```python
from build123d import *

# Parameters (mm, degrees)
EXTRUDE_1_DEPTH     = 15.5
EXTRUDE_2_DEPTH     = 3
FILLET_2_R          = 2
SKETCH_4_W          = 3
SKETCH_4_H          = 70
EXTRUDE_3_DEPTH     = 4
FILLET_3_R          = 1.5
CUT_EXTRUDE_3_DEPTH = 151.652746407
SKETCH_10_R         = 1.75
CUT_EXTRUDE_4_DEPTH = 164.099662783
SKETCH_9_R          = 1.75
CUT_EXTRUDE_5_DEPTH = 164.099662783


with BuildPart() as part:
    # 草图1 → 凸台-拉伸1 (new body)
    with BuildSketch(Plane(origin=(0, 0, 0), x_dir=(1, 0, 0), z_dir=(0, 1, 0))):
        with BuildLine():
            Line((-115, 85), (115, 85))
            ThreePointArc((115, 85), (118.535533906, 83.535533906), (120, 80))
            Line((120, 80), (120, -80))
            ThreePointArc((120, -80), (118.535533906, -83.535533906), (115, -85))
            Line((115, -85), (-115, -85))
            ThreePointArc((-115, -85), (-118.535533906, -83.535533906), (-120, -80))
            Line((-120, -80), (-120, 80))
            ThreePointArc((-120, 80), (-118.535533906, 83.535533906), (-115, 85))
        make_face()
        with BuildLine():
            Line((-112.5, 82.5), (112.5, 82.5))
            ThreePointArc((112.5, 82.5), (116.035533906, 81.035533906), (117.5, 77.5))
            Line((117.5, 77.5), (117.5, -77.5))
            ThreePointArc((117.5, -77.5), (116.035533906, -81.035533906), (112.5, -82.5))
            Line((112.5, -82.5), (-112.5, -82.5))
            ThreePointArc((-112.5, -82.5), (-116.035533906, -81.035533906), (-117.5, -77.5))
            Line((-117.5, -77.5), (-117.5, 77.5))
            ThreePointArc((-117.5, 77.5), (-116.035533906, 81.035533906), (-112.5, 82.5))
        make_face(mode=Mode.SUBTRACT)
    extrude(amount=EXTRUDE_1_DEPTH)

    # 草图3 → 凸台-拉伸2 (add)
    with BuildSketch(Plane(origin=(0, 15.5, 0), x_dir=(1, 0, 0), z_dir=(0, 1, 0))):
        with BuildLine():
            Line((-120, 80), (-120, -80))
            ThreePointArc((-120, -80), (-118.535533906, -83.535533906), (-115, -85))
            Line((-115, -85), (115, -85))
            ThreePointArc((115, -85), (118.535533906, -83.535533906), (120, -80))
            Line((120, -80), (120, 80))
            ThreePointArc((120, 80), (118.535533906, 83.535533906), (115, 85))
            Line((115, 85), (-115, 85))
            ThreePointArc((-115, 85), (-118.535533906, 83.535533906), (-120, 80))
        make_face()
    extrude(amount=EXTRUDE_2_DEPTH)

    # 圆角2
    fillet_2_edges = [part.edges().sort_by_distance(p)[0] for p in [
        (116.035533906, 15.5, -81.035533906),
        (0, 15.5, -82.5),
        (-116.035533906, 15.5, -81.035533906),
        (-117.5, 15.5, 0),
        (-116.035533906, 15.5, 81.035533906),
        (0, 15.5, 82.5),
        (116.035533906, 15.5, 81.035533906),
        (117.5, 15.5, 0),
        (-118.535533906, 18.5, -83.535533906),
        (-120, 18.5, 0),
        (-118.535533906, 18.5, 83.535533906),
        (0, 18.5, 85),
        (118.535533906, 18.5, 83.535533906),
        (120, 18.5, 0),
        (118.535533906, 18.5, -83.535533906),
        (0, 18.5, -85),
    ]]
    fillet(fillet_2_edges, radius=FILLET_2_R)

    # 草图4 → 凸台-拉伸3 (add)
    with BuildSketch(Plane.XZ):
        with Locations((-121.5, 0)):
            Rectangle(SKETCH_4_W, SKETCH_4_H)
        with Locations((121.5, 0)):
            Rectangle(SKETCH_4_W, SKETCH_4_H)
    extrude(amount=-EXTRUDE_3_DEPTH)

    # 圆角3
    fillet_3_edges = [part.edges().sort_by_distance(p)[0] for p in [
        (120, 4, 0),
        (-120, 4, 0),
        (-123, 4, 0),
        (123, 4, 0),
        (120, 2, -35),
        (123, 2, -35),
        (123, 2, 35),
        (120, 2, 35),
        (-120, 2, -35),
        (-123, 2, -35),
        (-123, 2, 35),
        (-120, 2, 35),
    ]]
    fillet(fillet_3_edges, radius=FILLET_3_R - 0.0001)  # a hair under: the kernel refuses the full size

    # 草图5 → 切除-拉伸3 (cut, through all)
    with BuildSketch(Plane(origin=(0, 18.5, 0), x_dir=(1, 0, 0), z_dir=(0, 1, 0))):
        with BuildLine():
            Line((80, 44.1), (-80, 44.1))
            ThreePointArc((-80, 44.1), (-87.778174593, 40.878174593), (-91, 33.1))
            Line((-91, 33.1), (-91, -33.1))
            ThreePointArc((-91, -33.1), (-87.778174593, -40.878174593), (-80, -44.1))
            Line((-80, -44.1), (80, -44.1))
            ThreePointArc((80, -44.1), (87.778174593, -40.878174593), (91, -33.1))
            Line((91, -33.1), (91, 33.1))
            ThreePointArc((91, 33.1), (87.778174593, 40.878174593), (80, 44.1))
        make_face()
    extrude(amount=-CUT_EXTRUDE_3_DEPTH, mode=Mode.SUBTRACT)

    # 草图10 → 切除-拉伸4 (cut, through all)
    with BuildSketch(Plane(origin=(0, 18.5, -20.5), x_dir=(1, 0, 0), z_dir=(0, -1, 0))):
        with Locations(Location((-92.325207, 65.878427, 0), (0, 0, 90))):
            Circle(SKETCH_10_R)
        with Locations(Location((92.325207, 65.878427, 0), (0, 0, 90))):
            Circle(SKETCH_10_R)
        with Locations(Location((92.325207, -24.878427, 0), (0, 0, 90))):
            Circle(SKETCH_10_R)
        with Locations(Location((-92.325207, -24.878427, 0), (0, 0, 90))):
            Circle(SKETCH_10_R)
    extrude(amount=CUT_EXTRUDE_4_DEPTH, mode=Mode.SUBTRACT)

    # 草图9 → 切除-拉伸5 (cut, through all)
    with BuildSketch(Plane(origin=(0, 18.5, -20.5), x_dir=(1, 0, 0), z_dir=(0, -1, 0))):
        with Locations(Location((-32.5, 69.55, 0), (0, 0, 90))):
            Circle(SKETCH_9_R)
        with Locations(Location((-95.99678, 42.5, 0), (0, 0, 90))):
            Circle(SKETCH_9_R)
        with Locations(Location((-32.5, -28.55, 0), (0, 0, 90))):
            Circle(SKETCH_9_R)
        with Locations(Location((-95.99678, -1.5, 0), (0, 0, 90))):
            Circle(SKETCH_9_R)
        with Locations(Location((32.5, -28.55, 0), (0, 0, 90))):
            Circle(SKETCH_9_R)
        with Locations(Location((95.99678, -1.5, 0), (0, 0, 90))):
            Circle(SKETCH_9_R)
        with Locations(Location((32.5, 69.55, 0), (0, 0, 90))):
            Circle(SKETCH_9_R)
        with Locations(Location((95.99678, 42.5, 0), (0, 0, 90))):
            Circle(SKETCH_9_R)
    extrude(amount=CUT_EXTRUDE_5_DEPTH, mode=Mode.SUBTRACT)


solid = part.part
```
Source: CAD feature listing. Evaluate the final solid. Frame: model axes, mm. A direction names the side the tool comes from. Give positions to 0.01 mm unless a question says otherwise; leave off trailing zeros. Write each loop counter-clockwise with the first axis right and the second up, starting at its lowest first coordinate (ties: lowest second). Pieces come first, ordered by that corner, then holes.
1. Section query D-D (z = -73). Return the cut outline in (x, y).
2. First-contact query: pin 1 (8 mm diameter, centred on y = 2, z = -52, fed in from -X); pin 2 (0.9 mm diameter, centred on y = 17.5, z = -2, fed in from +X); pin 3 (10 mm diameter, centred on y = 8, z = 29.5, fed in from +X); pin 4 (3 mm diameter, centred on x = -32.5, z = 49.05, fed in from +Y). Flat tips, straight axial feed; report the tip coordinate or a pass-through.
3. Pull-direction query (X, two-part tool) for faces 1 (the face through (2, 8, -85)), 2 (the face through (-120, 10, -1)), 3 (the face through (2, 7, 82.5)), 4 (the face through (119, 8, -83)); classes: +X half, -X half, draft (parallel to the pull), parting line (faces both ways), or undercut.
4. Access query for faces 5 (the face through (-119, 8, 83)), 6 (the face through (117.5, 7, -1)), 7 (the face through (-87.692, 17.021, -40.963)). Directions: +Z, -Z, +X, -X, +Y, -Y. A direction counts if a zero-diameter tool reaches every point of the face in a straight line with its end or side. Return the directions, or none.
5. Material intervals for line 1 along Z through (x, y) = (-32.5, 16.3); line 2 along Z through (x, y) = (54.5, 2); line 3 along X through (y, z) = (11, -58), sorted ascending.
6. Section query B-B (y = 8.25). Return the cut outline in (x, z).
7. Section query C-C (z = 41). Return the cut outline in (x, y), then the cut area to 3 significant figures.
8. Section query A-A (x = -62). Return the cut outline in (y, z).
Output values:
1. outline: (-120, 0) - (-117.5, 0) - (-117.5, 13.5) arc R2 cw to (-115.5, 15.5) - (115.5, 15.5) arc R2 cw to (117.5, 13.5) - (117.5, 0) - (120, 0) - (120, 16.5) arc R2 ccw to (118, 18.5) - (-118, 18.5) arc R2 ccw to (-120, 16.5) - close
2. pin 1: stops at x = -120
2. pin 2: stops at x = 119.92
2. pin 3: stops at x = 122.91
2. pin 4: passes through
3. face 1: draft
3. face 2: -X half
3. face 3: undercut
3. face 4: +X half
4. face 5: +Z, -X, +Y, -Y
4. face 6: -Y
4. face 7: +Y, -Y
5. line 1: z = -85 to -50.8, -47.3 to -44.1, 44.1 to 47.3, 50.8 to 85
5. line 2: z = -85 to -82.5, 82.5 to 85
5. line 3: x = -120 to -117.5, 117.5 to 120
6. outline: (-120, -80) arc R5 ccw to (-115, -85) - (115, -85) arc R5 ccw to (120, -80) - (120, 80) arc R5 ccw to (115, 85) - (-115, 85) arc R5 ccw to (-120, 80) - close; hole (-117.5, -77.5) arc R5 ccw to (-112.5, -82.5) - (112.5, -82.5) arc R5 ccw to (117.5, -77.5) - (117.5, 77.5) arc R5 ccw to (112.5, 82.5) - (-112.5, 82.5) arc R5 ccw to (-117.5, 77.5) - close
7. outline: (-120, 0) - (-117.5, 0) - (-117.5, 13.5) arc R2 cw to (-115.5, 15.5) - (-87.65, 15.5) - (-87.65, 18.5) - (-118, 18.5) arc R2 ccw to (-120, 16.5) - close; (87.65, 15.5) - (115.5, 15.5) arc R2 cw to (117.5, 13.5) - (117.5, 0) - (120, 0) - (120, 16.5) arc R2 ccw to (118, 18.5) - (87.65, 18.5) - close
7. area: 272 mm2
8. outline: (0, -85) - (16.5, -85) arc R2 ccw to (18.5, -83) - (18.5, -44.1) - (15.5, -44.1) - (15.5, -80.5) arc R2 cw to (13.5, -82.5) - (0, -82.5) - close; (0, 82.5) - (13.5, 82.5) arc R2 cw to (15.5, 80.5) - (15.5, 44.1) - (18.5, 44.1) - (18.5, 83) arc R2 ccw to (16.5, 85) - (0, 85) - close
